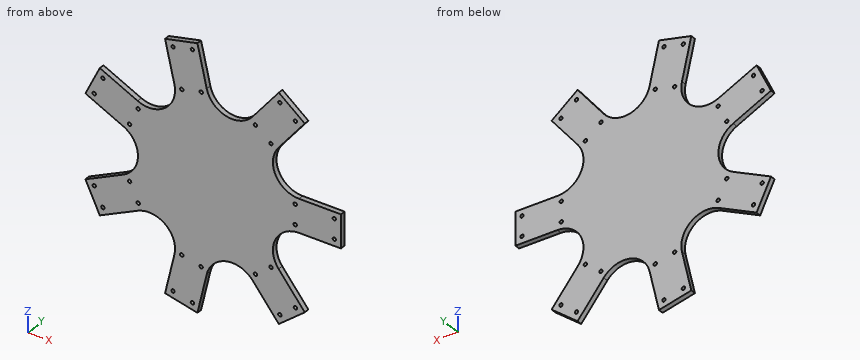
from build123d import *

# Parameters (mm, degrees)
SKETCH3_W           = 250
SKETCH3_H           = 63.5
SKETCH3_R           = 3.25
BOSS_EXTRUDE1_DEPTH = 10
CIRPATTERN1_COUNT   = 7
FILLET1_R           = 50


with BuildPart() as part:
    # Sketch3 → Boss-Extrude1 (new body)
    with BuildSketch(Plane(origin=(0, 0, 0), x_dir=(1, 0, 0), z_dir=(0, 1, 0))):
        with Locations((125, 0)):
            Rectangle(SKETCH3_W, SKETCH3_H)
        with Locations((162.3, 19.05)):
            Circle(SKETCH3_R, mode=Mode.SUBTRACT)
        with Locations((162.3, -19.05)):
            Circle(SKETCH3_R, mode=Mode.SUBTRACT)
        with Locations((237.3, 19.05)):
            Circle(SKETCH3_R, mode=Mode.SUBTRACT)
        with Locations((237.3, -19.05)):
            Circle(SKETCH3_R, mode=Mode.SUBTRACT)
    boss_extrude1 = extrude(amount=BOSS_EXTRUDE1_DEPTH)

    # CirPattern1: Boss-Extrude1 ×7 about axis
    cirpattern1_axis = Axis((0, 0, 0), (0, 1, 0))
    for i in range(1, CIRPATTERN1_COUNT):
        add(boss_extrude1.rotate(cirpattern1_axis, i * 360 / CIRPATTERN1_COUNT))

    # Fillet1
    fillet1_edges = [part.edges().sort_by_distance(p)[0] for p in [
        (65.929554341, 5, 31.75),
        (65.929554341, 5, -31.75),
        (16.283255204, 5, 71.341602418),
        (-45.624667219, 5, 57.211523112),
        (-73.176284653, 5, 0),
        (-45.624667219, 5, -57.211523112),
        (16.283255204, 5, -71.341602418),
    ]]
    fillet(fillet1_edges, radius=FILLET1_R)


solid = part.part
The listing builds one solid part. Answer for the finished solid, in the listing's coordinates (mm). Give positions to 0.01 mm unless a question says otherwise; leave off trailing zeros. Write each loop counter-clockwise with the first axis right and the second up, starting at its lowest first coordinate (ties: lowest second). Pieces come first, ordered by that corner, then holes. Notation, with made-up numbers: (-3, -14) - (44, -14) arc R31 ccw to (44, 18) - close; hole circle Ø2 at (36, 61). An arc over 180 degrees is marked (long way). One line per question, with ' | ' between items. Start each with the question number.
1. Given P1, Ø7.5, axis at x = 162.3, z = -19.05, coming from the -Y side; P2, Ø1, axis at x = 176, y = 6, coming from the -Z side; P3, Ø6, axis at x = 114.5, y = 4.5, coming from the +Z side; P4, Ø1.5, axis at y = 3.5, z = 46, coming from the +X side, each flat-ended and moving along its own axis, determine where each tip first touches the part or whether it passes through.
2. Section B-B, the plane x = -106.5 is taken. Determine the outline of the cut face in (y, z).
3. Straight lines are drawn through the part: line 1 (Z direction, x = 237.3, y = 6); line 2 (X direction, y = 3.75, z = 199.5); line 3 (X direction, y = 6.25, z = 172). For each, find the intervals that lie inside material, in ascending order.
4. Section A-A, the plane y = 5 is taken. Count the separate pieces of the cut face and the enclosed holes in it, then the cut area to 3 significant figures.
Result:
1) P1: stops at y = 0 | P2: stops at z = -179.81 | P3: stops at z = 198.26 | P4: stops at x = 135.58
2) outline: (0, -98.53) - (10, -98.53) - (10, 98.53) - (0, 98.53) - close
3) line 1: z = -31.75 to -22.3, -15.8 to 15.8, 22.3 to 31.75 | line 2: x = -78.1 to -12.97, 118.49 to 130.57, 135.55 to 150.8 | line 3: x = -71.82 to -6.69, 96.56 to 160.05, 165.65 to 177.78
4) separate pieces: 1 | enclosed holes: 28 | area: 112,000 mm2
